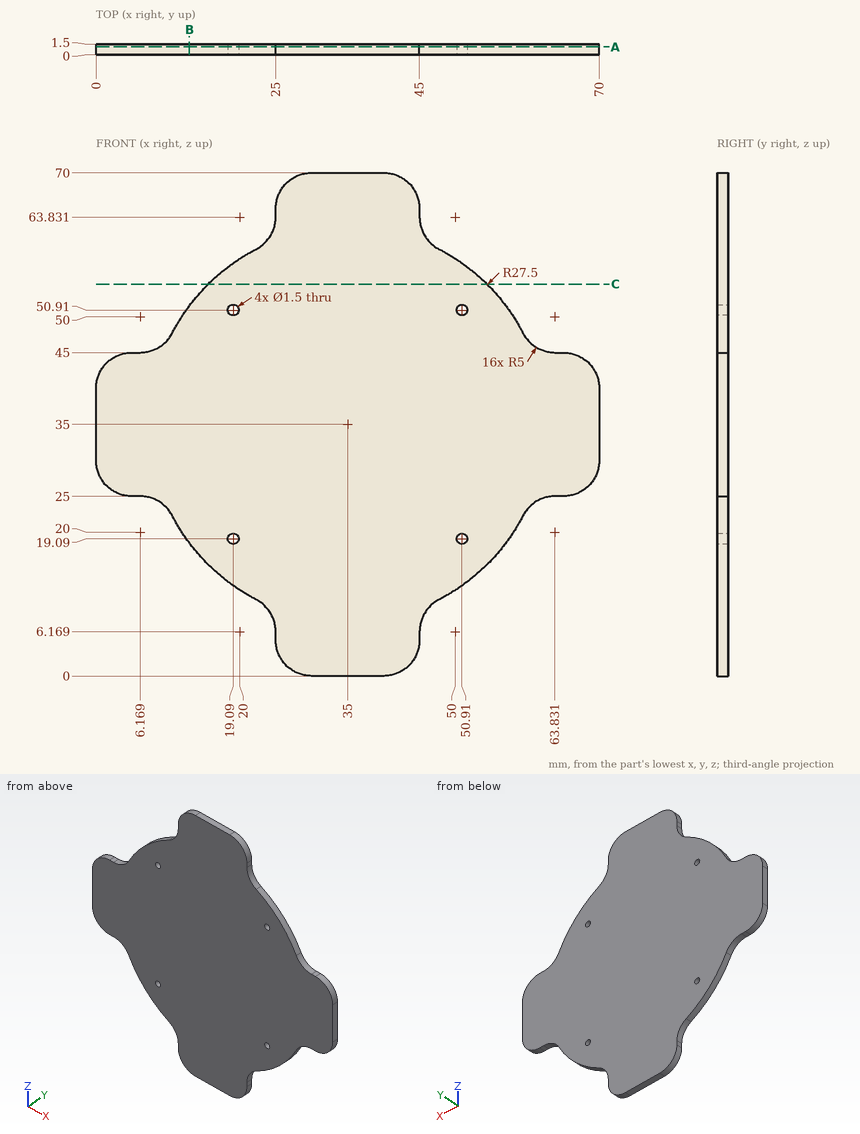
Source: three-view drawing plus pictorial views. Frame: mm from the lowest corner of the part. Round coordinates to 2 decimals unless told otherwise and drop trailing zeros. Loops run counter-clockwise (first coordinate to the right, second up) from the corner with the lowest first, then second, coordinate; pieces in that order, holes last.
1. Ray query, L1, parallel to Z at x = 50.5, y = 0.25 (1 decimal); L2, parallel to X at y = 0.4, z = 19 (1 decimal); L3, parallel to Z at x = 55, y = 0.55 (1 decimal). Return the intervals inside material, ascending.
2. Section query A-A on y = 1.1. Give the number of separate pieces and of enclosed holes in the cut face, and give its area (3 significant figures).
3. Contact query for flat-ended pins moving along their axis: pin 1 (0.9 mm diameter, centred on x = 19.09, z = 19.09, fed in from +Y); pin 2 (0.6 mm diameter, centred on y = 0.5, z = 64.5, fed in from +X). Output: stop coordinate, or through.
4. Section query C-C on z = 54.5. Output: boundary loops of the cut face in (x, y).
5. Section query B-B on x = 13. Output: boundary loops of the cut face in (y, z).
Answers below:
1. L1: z = 12.3 to 18.5, 19.7 to 50.3, 51.5 to 57.7
1. L2: x = 12.6 to 18.3, 19.8 to 50.2, 51.7 to 57.4
1. L3: z = 16.1 to 53.9
2. separate pieces: 1
2. enclosed holes: 4
2. area: 2,990 mm2
3. pin 1: passes through
3. pin 2: stops at x = 45
4. outline: (15.61, 0) - (54.39, 0) - (54.39, 1.5) - (15.61, 1.5) - close
5. outline: (0, 18.5) - (1.5, 18.5) - (1.5, 51.5) - (0, 51.5) - close
